Source: CAD feature listing. Evaluate the final solid. Frame: model axes, mm. Coordinates: 2 decimals unless noted, no trailing zeros. Loops run counter-clockwise (first coordinate to the right, second up) from the corner with the lowest first, then second, coordinate; pieces in that order, holes last. Notation, with made-up numbers: (69.25, -13) - (75.25, -13) arc R25 cw to (75.25, 25) - close; hole circle Ø8 at (42.25, -35). An arc over 180 degrees is marked (long way). Use one line per item in the form item = value. Start each with the question number.
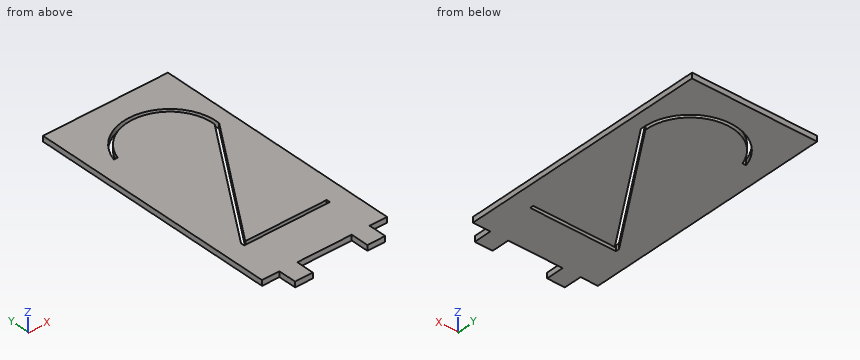
from build123d import *

# Parameters (mm, degrees)
SKIZZE1_W                        = 35
SKIZZE1_H                        = 75
AUFSATZ_LINEAR_AUSTRAGEN1_DEPTH  = 1.5
SKIZZE3_W                        = 15.25
SKIZZE3_H                        = 5
SKIZZE3_W_2                      = 4.875
SCHNITT_LINEAR_AUSTRAGEN12_DEPTH = 20
SCHNITT_LINEAR_AUSTRAGEN14_DEPTH = 1.5


with BuildPart() as part:
    # Skizze1 → Aufsatz-Linear austragen1 (new body)
    with BuildSketch(Plane.XY):
        with Locations((17.5, 37.5)):
            Rectangle(SKIZZE1_W, SKIZZE1_H)
    extrude(amount=AUFSATZ_LINEAR_AUSTRAGEN1_DEPTH)

    # Skizze3 → Schnitt-Linear austragen12 (cut)
    with BuildSketch(Plane.XY.offset(1.5)):
        with Locations((17.5, 2.5)):
            Rectangle(SKIZZE3_W, SKIZZE3_H)
        with Locations((32.5625, 2.5)):
            Rectangle(SKIZZE3_W_2, SKIZZE3_H)
        with Locations((2.4375, 2.5)):
            Rectangle(SKIZZE3_W_2, SKIZZE3_H)
    extrude(amount=-SCHNITT_LINEAR_AUSTRAGEN12_DEPTH, mode=Mode.SUBTRACT)

    # Skizze7 → Schnitt-Linear austragen14 (cut)
    with BuildSketch(Plane.XY.offset(1.5)):
        with BuildLine():
            Line((29.982770168, 54.357178796), (5.5, 18))
            Line((5.5, 18), (5.5, 17))
            Line((5.5, 17), (29.5, 17))
            Line((29.5, 17), (29.5, 18))
            Line((29.5, 18), (6.7, 18))
            Line((6.7, 18), (30.963924784, 54.032191031))
            ThreePointArc((30.963924784, 54.032191031), (20.317920223, 67.791686591), (5.520765623, 58.642623967))
            Line((5.520765623, 58.642623967), (6.566221507, 58.642623967))
            ThreePointArc((6.566221507, 58.642623967), (20.16023333, 66.803956623), (29.982770168, 54.357178796))
        make_face()
    extrude(amount=-SCHNITT_LINEAR_AUSTRAGEN14_DEPTH, mode=Mode.SUBTRACT)


solid = part.part
(1) Cut plane B-B, the plane y = 28. Output: boundary loops of the cut face in (x, z).
(2) Material intervals for line 1 (X direction, y = 4, z = 0.25) (3 decimals); line 2 (Y direction, x = 8, z = 1.25); line 3 (Y direction, x = 21, z = 1.35), sorted ascending.
(3) Cut plane C-C, the plane x = 11. Output: boundary loops of the cut face in (y, z).
(4) Contact query for a flat-ended pin moving along its axis: pin 1 (0.8 mm diameter, centred on x = 31.5, z = 1, fed in from -Y). Output: stop coordinate, or through.
(5) Cut plane D-D, the plane y = 60. Output: boundary loops of the cut face in (x, z).
(6) Cut plane A-A, the plane z = 0.85. Output: boundary loops of the cut face in (x, y) (3 decimals).
Recorded:
q1.outline = (0, 0) - (12.23, 0) - (12.23, 1.5) - (0, 1.5) - close; (13.43, 0) - (35, 0) - (35, 1.5) - (13.43, 1.5) - close
q2.line_1 = 4.875 to 9.875, 25.125 to 30.125
q2.line_2 = 0 to 17, 18 to 19.93, 21.71 to 61.63, 63.31 to 75
q2.line_3 = 5 to 17, 18 to 39.24, 41.02 to 66.62, 67.65 to 75
q3.outline = (5, 0) - (17, 0) - (17, 1.5) - (5, 1.5) - close; (18, 0) - (24.39, 0) - (24.39, 1.5) - (18, 1.5) - close; (26.17, 0) - (64.75, 0) - (64.75, 1.5) - (26.17, 1.5) - close; (65.95, 0) - (75, 0) - (75, 1.5) - (65.95, 1.5) - close
q4.pin_1 = 5
q5.outline = (0, 0) - (6, 0) - (6, 1.5) - (0, 1.5) - close; (7.09, 0) - (28.91, 0) - (28.91, 1.5) - (7.09, 1.5) - close; (30, 0) - (35, 0) - (35, 1.5) - (30, 1.5) - close
q6.outline = (0, 5) - (4.875, 5) - (4.875, 0) - (9.875, 0) - (9.875, 5) - (25.125, 5) - (25.125, 0) - (30.125, 0) - (30.125, 5) - (35, 5) - (35, 75) - (0, 75) - close; hole (5.5, 17) - (29.5, 17) - (29.5, 18) - (6.7, 18) - (30.964, 54.032) arc R13 ccw to (5.521, 58.643) - (6.566, 58.643) arc R12 cw to (29.983, 54.357) - (5.5, 18) - close
